The model under review builds one solid part; all positions refer to its coordinate system, in mm. Round coordinates to 2 decimals unless told otherwise and drop trailing zeros. Return JSON: item names as keys, results as strings.
Autodesk Inventor part; units mm, degrees
ref_plane "YZ Plane" through (0, 0, 0) normal (1, 0, 0) x (0, 1, 0)
ref_plane "XZ Plane" through (0, 0, 0) normal (0, 1, 0) x (-1, 0, 0)
ref_plane "XY Plane" through (0, 0, 0) normal (0, 0, 1) x (1, 0, 0)
sketch "Sketch1" plane through (0, 0, 0) normal (0, 1, 0) x (-1, 0, 0)
  line L0 (0, -102.1042) -> (0, 102.1042) construction
  line L1 (37.5532, 0) -> (-37.5532, 0) construction
  line L2 (500, 500) -> (-500, 500)
  line L3 (-500, 500) -> (-500, -500)
  line L4 (-500, -500) -> (500, -500)
  line L5 (500, -500) -> (500, 500)
  circle A0 centre (0, 0) radius 25
  dimension "d0" = 1000
  dimension "d1" = 1000
  dimension "d2" = 50
extrude "Extrusion1" add sketch "Sketch1" along normal blind 20
sketch "Sketch3" plane through (0, 20, 0) normal (0, 1, 0) x (1, 0, 0)
  line L0 (464.3817, -39.9852) -> (0, 0) construction
  line L1 (0, 0) -> (445.1648, -138.1214) construction
  line L2 (423.7332, -194.1633) -> (0, 0) construction
  line L3 (360.2723, -295.7246) -> (0, 0) construction
  line L4 (289.0138, -365.6778) -> (0, 0) construction
  line L5 (389.8771, -255.4312) -> (0, 0) construction
  line L6 (326.5218, -332.615) -> (0, 0) construction
  line L7 (230.9911, -404.8361) -> (0, 0) construction
  line L8 (139.32, -444.7911) -> (0, 0) construction
  line L9 (41.2359, -464.2723) -> (0, 0) construction
  line L10 (464.3817, -39.9852) -> (445.1648, -138.1214) construction
  line L11 (445.1648, -138.1214) -> (423.7332, -194.1633) construction
  line L12 (423.7332, -194.1633) -> (389.8771, -255.4312) construction
  line L13 (389.8771, -255.4312) -> (360.2723, -295.7246) construction
  line L14 (360.2723, -295.7246) -> (326.5218, -332.615) construction
  line L15 (326.5218, -332.615) -> (289.0138, -365.6778) construction
  line L16 (289.0138, -365.6778) -> (230.9911, -404.8361) construction
  line L17 (230.9911, -404.8361) -> (139.32, -444.7911) construction
  line L18 (139.32, -444.7911) -> (41.2359, -464.2723) construction
  line L19 (-58.7462, -462.3831) -> (0, 0) construction
  line L20 (-156.0243, -439.2102) -> (0, 0) construction
  line L21 (-200, -421.0098) -> (0, 0) construction
  line L22 (41.2359, -464.2723) -> (-58.7462, -462.3831) construction
  line L23 (-58.7462, -462.3831) -> (-156.0243, -439.2102) construction
  line L24 (-200, -421.0098) -> (-156.0243, -439.2102) construction
  line L25 (500, 500) -> (-500, 500)
  line L26 (500, -500) -> (500, 500)
  line L27 (-16.3542, 0) -> (16.3542, 0) construction
  line L28 (0, 9.5055) -> (0, -9.5055) construction
  line L29 (-500, -500) -> (500, -500)
  line L30 (-466.1, -260) -> (-466.1, -360) construction
  line L31 (-500, 500) -> (-500, -500) construction
  line L32 (-466.1, -260) -> (-466.1, -160) construction
  line L33 (-466.1, -160) -> (-466.1, -60) construction
  line L34 (-464.3817, 39.9852) -> (0, 0) construction
  line L35 (-445.1648, 138.1214) -> (0, 0) construction
  circle A0 centre (0, 0) radius 25 construction
  line L36 (-423.7332, 194.1633) -> (0, 0) construction
  line L37 (0, 0) -> (-389.8771, 255.4312) construction
  line L38 (-360.2723, 295.7246) -> (0, 0) construction
  line L39 (-326.5218, 332.615) -> (0, 0) construction
  line L40 (0, 0) -> (-289.0138, 365.6778) construction
  line L41 (-230.9911, 404.8361) -> (0, 0) construction
  line L42 (-139.32, 444.7911) -> (0, 0) construction
  line L43 (-41.2359, 464.2723) -> (0, 0) construction
  line L44 (-466.1, -60) -> (-464.3817, 39.9852) construction
  line L45 (-464.3817, 39.9852) -> (-445.1648, 138.1214) construction
  line L46 (-445.1648, 138.1214) -> (-423.7332, 194.1633) construction
  line L47 (-423.7332, 194.1633) -> (-389.8771, 255.4312) construction
  line L48 (-389.8771, 255.4312) -> (-360.2723, 295.7246) construction
  line L49 (-360.2723, 295.7246) -> (-326.5218, 332.615) construction
  line L50 (-326.5218, 332.615) -> (-289.0138, 365.6778) construction
  line L51 (-289.0138, 365.6778) -> (-230.9911, 404.8361) construction
  line L52 (-230.9911, 404.8361) -> (-139.32, 444.7911) construction
  line L53 (-139.32, 444.7911) -> (-41.2359, 464.2723) construction
  line L54 (58.7462, 462.3831) -> (0, 0) construction
  line L55 (156.0243, 439.2102) -> (0, 0) construction
  line L56 (200, 421.0098) -> (0, 0) construction
  line L57 (58.7462, 462.3831) -> (-41.2359, 464.2723) construction
  line L58 (58.7462, 462.3831) -> (156.0243, 439.2102) construction
  line L59 (156.0243, 439.2102) -> (200, 421.0098) construction
  point P0 (466.1, 360)
  point P1 (466.1, 260)
  point P2 (466.1, 160)
  point P3 (466.1, 60)
  dimension "d62" = 100
  dimension "d63" = 100
  dimension "d64" = 100
  dimension "d66" = 466.1
  dimension "d67" = 100
  dimension "d68" = 100
  dimension "d69" = 60
  dimension "d70" = 70
  dimension "d71" = 50
  dimension "d72" = 70
  dimension "d73" = 100
  dimension "d76" = 140
  dimension "d77" = 33.9
  dimension "d78" = 700
  dimension "d79" = 140
  dimension "d80" = 100
  dimension "d82" = 33.9
  dimension "d84" = 60
  dimension "d85" = 70
  dimension "d86" = 50
  dimension "d87" = 70
  dimension "d88" = 100
  dimension "d89" = 700
hole "Hole2" at (-200, 20, 421.0098) at (-156.0243, 20, 439.2102) at (-58.7462, 20, 462.3831) at (41.2359, 20, 464.2723) at (139.32, 20, 444.7911) at (230.9911, 20, 404.8361) at (289.0138, 20, 365.6778) at (326.5218, 20, 332.615) at (360.2723, 20, 295.7246) at (389.8771, 20, 255.4312) at (423.7332, 20, 194.1633) at (445.1648, 20, 138.1214) at (464.3817, 20, 39.9852) at (466.1, 20, -60) at (466.1, 20, -160) at (466.1, 20, -260) at (466.1, 20, -360) at (-466.1, 20, 360) at (-466.1, 20, 260) at (-466.1, 20, 160) at (-466.1, 20, 60) at (-464.3817, 20, -39.9852) at (-445.1648, 20, -138.1214) at (-423.7332, 20, -194.1633) at (-389.8771, 20, -255.4312) at (-360.2723, 20, -295.7246) at (-326.5218, 20, -332.615) at (-289.0138, 20, -365.6778) at (-230.9911, 20, -404.8361) at (-139.32, 20, -444.7911) at (-41.2359, 20, -464.2723) at (58.7462, 20, -462.3831) at (156.0243, 20, -439.2102) at (200, 20, -421.0098) direction (0, -1, 0) diameter 5.5 end through all
sketch "Sketch4" plane through (0, 20, 0) normal (0, 1, 0) x (1, 0, 0)
  line L0 (500, -500) -> (500, 500)
  line L1 (-500, 500) -> (-500, -500)
  line L2 (-500, -500) -> (500, -500)
  line L3 (500, 500) -> (-500, 500)
  line L4 (-360, 220) -> (-360, 77.5) construction
  line L5 (-360, 77.5) -> (-360, -65) construction
  line L6 (-360, -65) -> (-360, -207.5) construction
  line L7 (-360, -207.5) -> (-360, -350) construction
  line L8 (360, 350) -> (360, 207.5) construction
  line L9 (360, 207.5) -> (360, 65) construction
  line L10 (360, 65) -> (360, -77.5) construction
  line L11 (360, -77.5) -> (360, -220) construction
  line L12 (310, -280) -> (155, -280) construction
  line L13 (155, -280) -> (0, -280) construction
  line L14 (0, -280) -> (-155, -280) construction
  line L15 (-155, -280) -> (-310, -280) construction
  line L16 (-310, 280) -> (-155, 280) construction
  line L17 (-155, 280) -> (0, 280) construction
  line L18 (0, 280) -> (155, 280) construction
  line L19 (155, 280) -> (310, 280) construction
  line L20 (0, 7.0345) -> (0, -7.0345) construction
  line L21 (-9.8826, 0) -> (9.8826, 0) construction
  point P0 (0, 0)
  point P1 (-45, 65)
  point P2 (-45, -65)
  point P3 (45, -65)
  point P4 (45, 65)
  point P5 (0, 0)
  dimension "d42" = 140
  dimension "d43" = 140
  dimension "d44" = 150
  dimension "d45" = 150
  dimension "d46" = 570
  dimension "d47" = 570
  dimension "d55" = 220
  dimension "d56" = 220
  dimension "d57" = 50
  dimension "d58" = 50
  dimension "d59" = 90
  dimension "d60" = 130
hole "Hole3" at (360, 20, -350) at (360, 20, -207.5) at (360, 20, 77.5) at (360, 20, 220) at (360, 20, -65) at (-360, 20, 350) at (-360, 20, 207.5) at (-360, 20, 65) at (-360, 20, -220) at (-360, 20, -77.5) at (-310, 20, -280) at (-155, 20, -280) at (0, 20, -280) at (155, 20, -280) at (310, 20, -280) at (310, 20, 280) at (155, 20, 280) at (0, 20, 280) at (-155, 20, 280) at (-310, 20, 280) at (-45, 20, -65) at (45, 20, -65) at (-45, 20, 65) at (45, 20, 65) direction (0, -1, 0) diameter 5.5 end through all countersink diameter 10.4 countersink angle 90
properties part number "groundPlateWoodV1" material "PMMA Plastic"
(1) Mouldability with a two-part tool opening along Z and no side actions: class faces 1 (the cylindrical face through (-23.846, 9.86, -7.509)), 2 (the flat face through (118, 0, 7)) as released by +Z, released by -Z, zero draft, split by the parting line, or undercut.
Filled in:
{"face 1": "undercut", "face 2": "zero draft"}
(2) Clearance check with flat-ended pins moving along their axes: pin 1 Ø10 at (x, z) = (-267, -230.5) entering from -Y; pin 2 Ø6.5 at (x, z) = (-360, 207.5) entering from +Y; pin 3 Ø7 at (x, z) = (-310, -280) entering from +Y. State where each tip first meets the part, or that it passes through.
Filled in:
{"pin 1": "stops at y = 0", "pin 2": "stops at y = 18.05", "pin 3": "stops at y = 18.3"}
(3) Wall thickness on line 1 (Z direction, x = 44.5, y = 10); line 2 (X direction, y = 5.25, z = -280); line 3 (X direction, y = 10, z = 207.5): over which ranges is each line inside the solid? List them lowest first.
Filled in:
{"line 1": "z = -500 to -67.7, -62.3 to 62.3, 67.7 to 500", "line 2": "x = -500 to -312.75, -307.25 to -157.75, -152.25 to -2.75, 2.75 to 152.25, 157.75 to 307.25, 312.75 to 500", "line 3": "x = -500 to -362.75, -357.25 to 500"}
